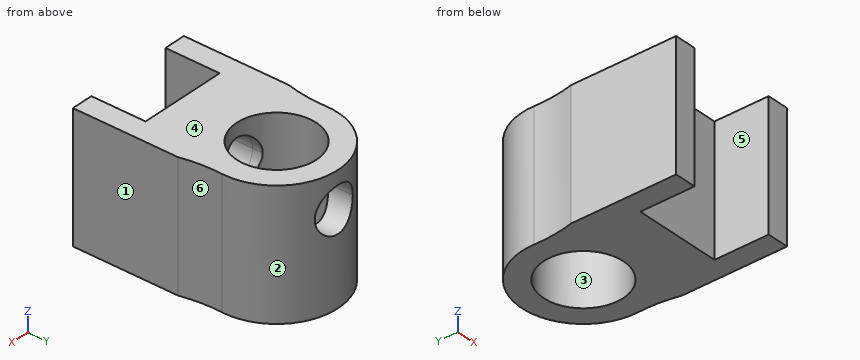
```python
from build123d import *
from build123d import SkipClean  # not in build123d's __all__

# Parameters (mm, degrees)
F1_DEPTH    = 17.5
F2_DEPTH    = 9
F3_T4_DEPTH = 24.2978178738
F3_T9_DEPTH = 24.2978178738
F5_DEPTH    = 8.5
F6_DEPTH    = 25
F7_DEPTH    = 5
F8_DEPTH    = 25


# Not quite as in the source:
# - a fillet or chamfer that OpenCascade refuses, or shapes differently, is made with other operations: its cross-section is extruded or revolved along the edge and cut away or added
# - after a boolean that leaves OpenCascade's solid faulty, fix() repairs it
# - a feature names something its author has since deleted; it is built from what else it names


with BuildPart() as f1:
    # F0 (on Top) → F1 (new body)
    with BuildSketch(Plane.XY):
        Polygon((-6.05, -13), (-6.05, -5.9705527382), (-9.05, -5.9705527382), (-9.05, -20.5), (-6.05, -20.5), align=None)
        with BuildLine():
            Line((0, -13), (0, -8.5))
            ThreePointArc((0, -8.5), (-3.2787422684, -7.842183952), (-6.05, -5.9705527382))
            Line((-6.05, -5.9705527382), (-6.05, -13))
            Line((-6.05, -13), (0, -13))
        make_face()
        with BuildLine():
            ThreePointArc((6.05, -5.9705527382), (3.2787422684, -7.842183952), (0, -8.5))
            Line((0, -8.5), (0, -13))
            Line((0, -13), (6.05, -13))
            Line((6.05, -13), (6.05, -5.9705527382))
        make_face()
        Polygon((9.05, -5.9705527382), (6.05, -5.9705527382), (6.05, -13), (6.05, -20.5), (9.05, -20.5), align=None)
    extrude(amount=F1_DEPTH)

    # F0 (on Top) → F2 (join)
    with BuildSketch(Plane.XY):
        with BuildLine():
            Line((-6.05, -5.9705527382), (0, -5.9705527382))
            Line((0, -5.9705527382), (6.05, -5.9705527382))
            Line((6.05, -5.9705527382), (6.05, 5.9705527382))
            ThreePointArc((6.05, 5.9705527382), (0, 8.5), (-6.05, 5.9705527382))
            Line((-6.05, 5.9705527382), (-6.05, -5.9705527382))
        make_face()
        with BuildLine():
            ThreePointArc((0, -5.5), (-3.8890872965, 3.8890872965), (5.5, 0))
            ThreePointArc((5.5, 0), (3.8890872965, -3.8890872965), (0, -5.5))
        make_face(mode=Mode.SUBTRACT)
        with BuildLine():
            Line((6.05, 5.9705527382), (6.05, -5.9705527382))
            ThreePointArc((6.05, -5.9705527382), (7.8636823435, -3.2268405601), (8.5, 0))
            ThreePointArc((8.5, 0), (7.8636823435, 3.2268405601), (6.05, 5.9705527382))
        make_face()
        with BuildLine():
            ThreePointArc((-6.05, 5.9705527382), (-8.5, 0), (-6.05, -5.9705527382))
            Line((-6.05, -5.9705527382), (-6.05, 5.9705527382))
        make_face()
        with BuildLine():
            Line((0, -8.5), (0, -5.9705527382))
            Line((0, -5.9705527382), (-6.05, -5.9705527382))
            ThreePointArc((-6.05, -5.9705527382), (-3.2787422684, -7.842183952), (0, -8.5))
        make_face()
        with BuildLine():
            Line((6.05, -5.9705527382), (0, -5.9705527382))
            Line((0, -5.9705527382), (0, -8.5))
            ThreePointArc((0, -8.5), (3.2787422684, -7.842183952), (6.05, -5.9705527382))
        make_face()
    extrude(amount=F2_DEPTH)

    # F3: fillet of radius 20 on 4 edges, made by hand


with BuildPart() as f3_tool2:
    # F3_s3 → F3_t4 (new body)
    with BuildSketch(Plane.XY):
        with BuildLine():
            ThreePointArc((-9.05, -5.9705527382), (-8.5724849096, -3.1850150396), (-8.492373898, -0.3599799676))
            ThreePointArc((-8.492373898, -0.3599799676), (-7.7935737214, -3.3926698409), (-6.05, -5.9705527382))
            Line((-6.05, -5.9705527382), (-9.05, -5.9705527382))
        make_face()
    extrude(amount=F3_T4_DEPTH)

    split(bisect_by=Plane.XY.offset(17.5), keep=Keep.BOTTOM)


with BuildPart() as f1_1:
    add(f1.part, clean=False)

    # F3_t1: union F3_tool2
    add(f3_tool2.part)


with BuildPart() as f3_tool7:
    # F3_s8 → F3_t9 (new body)
    with BuildSketch(Plane.XY):
        with BuildLine():
            ThreePointArc((9.05, -5.9705527382), (8.5724849096, -3.1850150396), (8.492373898, -0.3599799676))
            ThreePointArc((8.492373898, -0.3599799676), (7.7935737214, -3.3926698409), (6.05, -5.9705527382))
            Line((6.05, -5.9705527382), (9.05, -5.9705527382))
        make_face()
    extrude(amount=F3_T9_DEPTH)

    split(bisect_by=Plane.XY.offset(17.5), keep=Keep.BOTTOM)


with BuildPart() as f1_2:
    add(f1_1.part, clean=False)

    # F3_t6: union F3_tool7
    add(f3_tool7.part)

    # F5 (add, through all): a face of the model
    f5_faces = [f1_2.faces().sort_by_distance(p)[0] for p in [
        (0, -8.2595836944, 9),
    ]]
    extrude(f5_faces, amount=F5_DEPTH)

    # F4 (on face) → F6 (cut)
    with BuildSketch(Plane(origin=(0, -5.9705527382, 0), x_dir=(-1, 0, 0), z_dir=(0, 1, 0))):
        with BuildLine():
            ThreePointArc((3.1, 12.5), (2.1920310217, 14.6920310217), (0, 15.6))
            ThreePointArc((0, 15.6), (-2.1920310217, 10.3079689783), (3.1, 12.5))
        make_face()
        with BuildLine():
            ThreePointArc((1.6, 12.5), (-1.1313708499, 11.3686291501), (0, 14.1))
            ThreePointArc((0, 14.1), (1.1313708499, 13.6313708499), (1.6, 12.5))
        make_face(mode=Mode.SUBTRACT)
        with BuildLine():
            ThreePointArc((1.6, 12.5), (1.1313708499, 13.6313708499), (0, 14.1))
            ThreePointArc((0, 14.1), (-1.1313708499, 11.3686291501), (1.6, 12.5))
        make_face()
    extrude(amount=F6_DEPTH, mode=Mode.SUBTRACT)

    # F4 (on face) → F7 (cut)
    with BuildSketch(Plane(origin=(0, -5.9705527382, 0), x_dir=(-1, 0, 0), z_dir=(0, 1, 0))):
        with BuildLine():
            ThreePointArc((3.1, 12.5), (2.1920310217, 14.6920310217), (0, 15.6))
            ThreePointArc((0, 15.6), (-2.1920310217, 10.3079689783), (3.1, 12.5))
        make_face()
        with BuildLine():
            ThreePointArc((1.6, 12.5), (-1.1313708499, 11.3686291501), (0, 14.1))
            ThreePointArc((0, 14.1), (1.1313708499, 13.6313708499), (1.6, 12.5))
        make_face(mode=Mode.SUBTRACT)
    with SkipClean():  # cleaning this boolean's faces spoils the solid; the shape is the same uncleaned
        extrude(amount=-F7_DEPTH, mode=Mode.SUBTRACT)

    # F4 (on face) → F8 (cut)
    with BuildSketch(Plane(origin=(0, -5.9705527382, 0), x_dir=(-1, 0, 0), z_dir=(0, 1, 0))):
        with BuildLine():
            ThreePointArc((1.6, 12.5), (1.1313708499, 13.6313708499), (0, 14.1))
            ThreePointArc((0, 14.1), (-1.1313708499, 11.3686291501), (1.6, 12.5))
        make_face()
    extrude(amount=-F8_DEPTH, mode=Mode.SUBTRACT)

    add(f1_2.part.fix(), mode=Mode.REPLACE)


solid = f1_2.part
```
Work out the finished part from the listing and answer in its coordinate system (mm). Face numbers are marked on the shaded views. A direction names the side the tool comes from. Round coordinates to 2 decimals unless told otherwise and drop trailing zeros. Write each loop counter-clockwise with the first axis right and the second up, starting at its lowest first coordinate (ties: lowest second). Pieces come first, ordered by that corner, then holes. Notation, with made-up numbers: (-6, 40.5) - (39, 40.5) arc R15 ccw to (39, 66.5) - close; hole circle Ø6 at (77.25, 12). An arc over 180 degrees is marked (long way). Return JSON: item names as keys, results as strings. Group by question number.
Q1. The mould has two halves that part along X. Classify the marked faces 1, 2 and 3: released by +X, released by -X, zero draft, split by the parting line, or undercut.
Q2. The part is cut by section C-C on x = 4. Write down the section's boundary in (y, z), then the cut area to 3 significant figures.
Q3. The part is cut by section B-B on z = 2. Write down the section's boundary in (x, y).
Q4. The part is cut by section A-A on y = -15.75. Write down the section's boundary in (x, z).
Q5. Each of these flat-tipped pins is pushed along its axis until it touches: pin 1 Ø10 at (x, z) = (-5, 14.5) entering from -Y; pin 2 Ø1.9 at (x, z) = (0, 12.5) entering from +Y; pin 3 Ø10 at (y, z) = (2.5, 7) entering from +X; pin 4 Ø8 at (x, z) = (0, 12.5) entering from -Y. Where does it stop, or does it pass through?
Q6. The part is cut by section D-D on y = -6.75. Write down the section's boundary in (x, z), then the cut area to 3 significant figures.
Q7. For the marked faces 4, 5 and 6, determine the directions among +Z, -Z, +X, -X, +Y, -Y from which every point of the face is accessible in a straight line to the end or side of a thin tool.
Q8. Find the intervals of material crossed by L1, parallel to X at y = -17.5, z = 5; L2, parallel to Z at x = 0, y = -12.2; L3, parallel to Y at x = 0, z = 7, in increasing order.
Solved:
{
 "1": {"face 1": "released by +X", "face 2": "split by the parting line", "face 3": "undercut"},
 "2": {"outline": "(-13, 0) - (-3.77, 0) - (-3.77, 17.5) - (-13, 17.5) - close; (3.77, 0) - (7.5, 0) - (7.5, 17.5) - (3.77, 17.5) - close", "area": "227 mm²"},
 "3": {"outline": "(-9.05, -20.5) - (-6.05, -20.5) - (-6.05, -13) - (6.05, -13) - (6.05, -20.5) - (9.05, -20.5) - (9.05, -5.97) arc R20 cw to (8.49, -0.36) arc R8.5 ccw (long way) to (-8.49, -0.36) arc R20 cw to (-9.05, -5.97) - close; hole circle Ø11 at (0, 0)"},
 "4": {"outline": "(-9.05, 0) - (-6.05, 0) - (-6.05, 17.5) - (-9.05, 17.5) - close; (6.05, 0) - (9.05, 0) - (9.05, 17.5) - (6.05, 17.5) - close"},
 "5": {"pin 1": "y = -20.5", "pin 2": "through", "pin 3": "x = 8.52", "pin 4": "y = -13"},
 "6": {"outline": "(-9.05, 0) - (9.05, 0) - (9.05, 17.5) - (-9.05, 17.5) - close; hole circle Ø6.2 at (0, 12.5)", "area": "287 mm²"},
 "7": {"face 4": "+Z, +X, -X, +Y, -Y", "face 5": "+Z, -Z, -Y", "face 6": "+Z, -Z, +X"},
 "8": {"L1": "-9.05 to -6.05, 6.05 to 9.05", "L2": "0 to 10.9, 14.1 to 17.5", "L3": "-13 to -5.5, 5.5 to 8.5"}
}
